Work out the finished part from the listing and answer in its coordinate system (mm). Face numbers are marked on the shaded views. A direction names the side the tool comes from. Round coordinates to 2 decimals unless told otherwise and drop trailing zeros. Loops run counter-clockwise (first coordinate to the right, second up) from the corner with the lowest first, then second, coordinate; pieces in that order, holes last. Notation, with made-up numbers: M -19.75,-25 L 23.25,-25 A27 cw 23.25,5 Z; hole C 72.5,84 d3. An arc over 180 degrees is marked long. One line per item, written item: value.
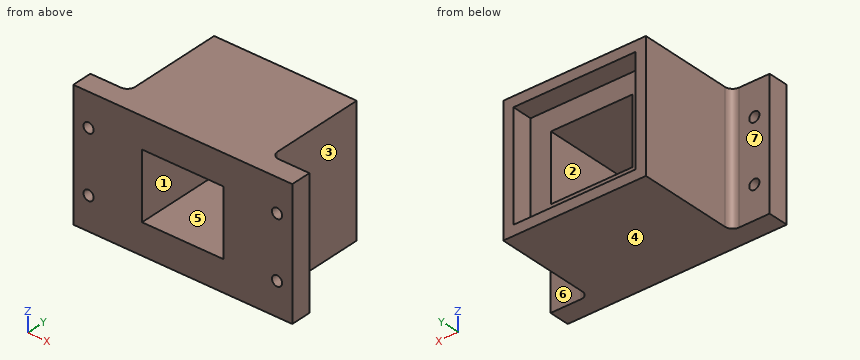
```python
from build123d import *

# Parameters (mm, degrees)
SKETCH1_W               = 56
SKETCH1_H               = 50
BOSS_EXTRUDE1_DEPTH     = 48
SKETCH3_W               = 48
SKETCH3_H               = 42
CUT_EXTRUDE1_DEPTH      = 8
SKETCH4_W               = 15
SKETCH4_H               = 8
BOSS_EXTRUDE2_DEPTH     = 50
FILLET1_R               = 3
CUT_EXTRUDE2_DEPTH      = 64.827893589
CUT_EXTRUDE2_DEPTH_BACK = 64.827893589
SKETCH5_W               = 32
SKETCH5_H               = 26
CUT_EXTRUDE3_DEPTH      = 64.827893589
CUT_EXTRUDE3_DEPTH_BACK = 64.827893589
SKETCH6_R               = 2


with BuildPart() as part:
    # Sketch1 → Boss-Extrude1 (new body)
    with BuildSketch(Plane(origin=(0, 0, 0), x_dir=(1, 0, 0), z_dir=(0, 1, 0))):
        Rectangle(SKETCH1_W, SKETCH1_H)
    extrude(amount=BOSS_EXTRUDE1_DEPTH)

    # Sketch3 → Cut-Extrude1 (cut)
    with BuildSketch(Plane(origin=(0, 48, 0), x_dir=(1, 0, 0), z_dir=(0, 1, 0))):
        Rectangle(SKETCH3_W, SKETCH3_H)
    extrude(amount=-CUT_EXTRUDE1_DEPTH, mode=Mode.SUBTRACT)

    # Sketch4 → Boss-Extrude2 (add)
    with BuildSketch(Plane.XY.offset(25)):
        with Locations((-35.5, 4)):
            Rectangle(SKETCH4_W, SKETCH4_H)
        with Locations((35.5, 4)):
            Rectangle(SKETCH4_W, SKETCH4_H)
    extrude(amount=-BOSS_EXTRUDE2_DEPTH)

    # Fillet1
    fillet1_edges = [part.edges().sort_by_distance(p)[0] for p in [
        (-28, 8, 0),
        (28, 8, 0),
    ]]
    fillet(fillet1_edges, radius=FILLET1_R)

    # Sketch5 → Cut-Extrude2 (cut, two sides: drawn at the far end of the back side and taken through both)
    with BuildSketch(Plane(origin=(0, 40, 0), x_dir=(1, 0, 0), z_dir=(0, 1, 0)).offset(-CUT_EXTRUDE2_DEPTH_BACK)):
        Rectangle(SKETCH5_W, SKETCH5_H)
    extrude(amount=CUT_EXTRUDE2_DEPTH + CUT_EXTRUDE2_DEPTH_BACK, mode=Mode.SUBTRACT)

    # Sketch6 → Cut-Extrude3 (cut, two sides: drawn at the far end of the back side and taken through both)
    with BuildSketch(Plane(origin=(0, 8, 0), x_dir=(1, 0, 0), z_dir=(0, 1, 0)).offset(-CUT_EXTRUDE3_DEPTH_BACK)):
        with Locations(Location((-37, 12.079385962, 0), (0, 0, 180))):
            Circle(SKETCH6_R)
        with Locations(Location((-37, -12.079385962, 0), (0, 0, 180))):
            Circle(SKETCH6_R)
        with Locations((37, -12.079385962)):
            Circle(SKETCH6_R)
        with Locations((37, 12.079385962)):
            Circle(SKETCH6_R)
    extrude(amount=CUT_EXTRUDE3_DEPTH + CUT_EXTRUDE3_DEPTH_BACK, mode=Mode.SUBTRACT)


solid = part.part
```
1) Find section B-B (z = -7). Give the vertices of the cut face in (x, y).
Check values:
outline: M -43,0 L -16,0 L -16,40 L -24,40 L -24,48 L -28,48 L -28,11 A3 cw -31,8 L -43,8 Z; M 16,0 L 43,0 L 43,8 L 31,8 A3 cw 28,11 L 28,48 L 24,48 L 24,40 L 16,40 Z
2) Find section A-A (x = -37). Give the vertices of the cut face in (y, z).
Check values:
outline: M 0,-25 L 8,-25 L 8,-14.08 L 0,-14.08 Z; M 0,-10.08 L 8,-10.08 L 8,10.08 L 0,10.08 Z; M 0,14.08 L 8,14.08 L 8,25 L 0,25 Z
3) Find the intervals of material crossed by probe 1 along Z at (x, y) = (-37, 2.25); probe 2 along X at (y, z) = (39.5, 2); probe 3 along Z at (x, y) = (1, 37.5), in increasing order. Write a range as from..to.
Check values:
probe 1: -25..-14.08, -10.08..10.08, 14.08..25
probe 2: -28..-16, 16..28
probe 3: -25..-13, 13..25
4) The mould has two halves that part along X. Classify the marked faces 1, 2, 3 and 4: +X half, -X half, draft (parallel to the pull), parting line (faces both ways), or undercut.
Check values:
face 1: undercut
face 2: undercut
face 3: +X half
face 4: draft
5) Each of these flat-tipped pins is pushed along its axis until it touches: pin 1 (4 mm diameter, centred on y = 42, z = 6.5, fed in from -X); pin 2 (8 mm diameter, centred on y = 13, z = -1, fed in from +X); pin 3 (6 mm diameter, centred on y = 39.5, z = -14.5, fed in from +X); pin 4 (5 mm diameter, centred on x = 32, y = 24.5, fed in from -Z). Where does it stop, or does it pass through?
Check values:
pin 1: x = -28
pin 2: x = 28.76
pin 3: x = 28
pin 4: through
6) Find section D-D (z = -19.5). Give the vertices of the cut face in (x, y).
Check values:
outline: M -43,0 L 43,0 L 43,8 L 31,8 A3 cw 28,11 L 28,48 L 24,48 L 24,40 L -24,40 L -24,48 L -28,48 L -28,11 A3 cw -31,8 L -43,8 Z
7) Find section C-C (y = 19.5). Give the vertices of the cut face in (x, z).
Check values:
outline: M -28,-25 L 28,-25 L 28,25 L -28,25 Z; hole M -16,-13 L 16,-13 L 16,13 L -16,13 Z
8) For the marked faces 5, 6 and 7, determine the directions among +Z, -Z, +X, -X, +Y, -Y from which every point of the face is accessible in a straight line to the end or side of a thin tool.
Check values:
face 5: +Y, -Y
face 6: +Z, -Z, +X, +Y
face 7: +Z, -Z, -X, +Y
